Here's how the part is built. I have some questions about the finished solid (model axes, mm). Face numbers are marked on the shaded views. A direction names the side the tool comes from. Coordinates: 2 decimals unless noted, no trailing zeros. Write each loop counter-clockwise with the first axis right and the second up, starting at its lowest first coordinate (ties: lowest second). Pieces come first, ordered by that corner, then holes. Notation, with made-up numbers: (-8, 69.25) - (21, 69.25) arc R17 ccw to (21, 93.25) - close; hole circle Ø4 at (-28.5, 48). An arc over 180 degrees is marked (long way). Answer in a Markdown table with one row per item. Add a question column.
Item 1: If I drill on probe 1 along X at (y, z) = (13, -67); probe 2 along X at (y, z) = (25.75, -47); probe 3 along Z at (x, y) = (35, 24.5), over which ranges is the centre line in solid material (lowest first)? Write a range as from..to.
Item 2: I'm going to push flat-ended pins straight in: pin 1 (1.5 mm diameter, centred on x = 60.5, y = 16.5, fed in from -Z); pin 2 (12 mm diameter, centred on x = 5, z = -53, fed in from -Y); pin 3 (3 mm diameter, centred on x = 37.5, y = 9.5, fed in from -Z). Where does each tip first touch, or does it pass through?
Item 3: Which directions (+Z, -Z, +X, -X, +Y, -Y) give clear straight access to the entire face, cutting with the end or side of a thin tool? Please do the marked faces 4 and 5.
Item 4: Imagine slicing it at B-B (y = 1.75). Please give me the cut outline in (x, z).
Item 5: Imagine slicing it at C-C (x = 14). Please give me the cut outline in (y, z), plus the area to 3 significant figures.
Item 6: Imagine slicing it at A-A (z = -51). Please give me the cut outline in (x, y), plus the area to 3 significant figures.
Item 7: Imagine slicing it at D-D (z = -43). Please give me the cut outline in (x, y) (3 decimals).
Item 8: We'd pull the mould along X, two halves only. Please class the marked faces 1, 2 and 3: +X half, -X half, draft (parallel to the pull), parting line (faces both ways), or undercut.
from build123d import *

# Parameters (mm, degrees)
SKIZZE1_W                       = 95
SKIZZE1_H                       = 70
AUFSATZ_LINEAR_AUSTRAGEN1_DEPTH = 28.3
SCHNITT_LINEAR_AUSTRAGEN1_REACH = 123.35
SKIZZE2_W                       = 7.37
SKIZZE2_H                       = 3
SCHNITT_LINEAR_AUSTRAGEN2_DEPTH = 30
VERRUNDUNG1_R                   = 8.5
AUFSATZ_LINEAR_AUSTRAGEN3_DEPTH = 3
VERRUNDUNG2_R                   = 8


with BuildPart() as part:
    # Skizze1 → Aufsatz-Linear austragen1 (new body)
    with BuildSketch(Plane(origin=(0, 0, 0), x_dir=(1, 0, 0), z_dir=(0, 1, 0))):
        with Locations((47.5, 35)):
            Rectangle(SKIZZE1_W, SKIZZE1_H)
    extrude(amount=AUFSATZ_LINEAR_AUSTRAGEN1_DEPTH)

    # Skizze2 → Schnitt-Linear austragen1 (cut, up to next)
    with BuildSketch(Plane.XY, mode=Mode.PRIVATE) as schnitt_linear_austragen1_sk1:
        with Locations((58.855, 26.8)):
            Rectangle(SKIZZE2_W, SKIZZE2_H)
    schnitt_linear_austragen1_tool1 = extrude(schnitt_linear_austragen1_sk1.sketch, amount=-SCHNITT_LINEAR_AUSTRAGEN1_REACH, mode=Mode.PRIVATE) & part.part
    add(schnitt_linear_austragen1_tool1.solids().sort_by_distance((58.855, 26.8, 0))[0], mode=Mode.SUBTRACT)

    # Skizze4 → Schnitt-Linear austragen2 (cut)
    with BuildSketch(Plane(origin=(0, 0, -70), x_dir=(-1, 0, 0), z_dir=(0, 0, -1))):
        Polygon((-3.63, 0), (-71.13, 0), (-71.13, 3), (-66.63, 3), (-66.63, 28.3), (-49.63, 28.3), (-49.63, 3), (-43.63, 3), (-43.63, 28.3), (-26.63, 28.3), (-26.63, 3), (-20.63, 3), (-20.63, 28.3), (-3.63, 28.3), (-3.63, 3), (0, 3), (0, 0), align=None)
    extrude(amount=-SCHNITT_LINEAR_AUSTRAGEN2_DEPTH, mode=Mode.SUBTRACT)

    # Verrundung1
    verrundung1_edges = [part.edges().sort_by_distance(p)[0] for p in [
        (3.63, 15.65, -40),
        (20.63, 15.65, -40),
        (26.63, 15.65, -40),
        (43.63, 15.65, -40),
        (49.63, 15.65, -40),
        (66.63, 15.65, -40),
    ]]
    fillet(verrundung1_edges, radius=VERRUNDUNG1_R - 0.0001)  # a hair under: the kernel refuses the full size

    # Skizze5 → Aufsatz-Linear austragen3 (add)
    with BuildSketch(Plane.ZY):
        Polygon((0, 0), (-40, 0), (-40, 3), (-70, 3), (-70, 28.3), (0, 28.3), align=None)
    extrude(amount=AUFSATZ_LINEAR_AUSTRAGEN3_DEPTH)

    # Verrundung2
    verrundung2_edges = [part.edges().sort_by_distance(p)[0] for p in [
        (71.13, 1.5, -40),
    ]]
    fillet(verrundung2_edges, radius=VERRUNDUNG2_R)


solid = part.part
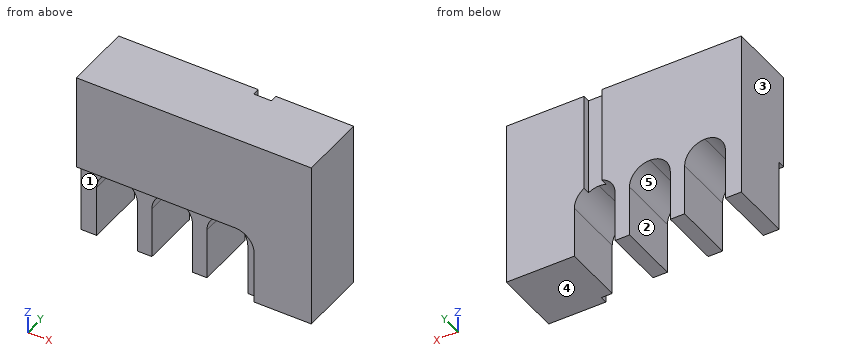
Here are the results:
| question | item | result |
|---|---|---|
| 1 | probe 1 | x = -3..3.63, 20.63..26.63, 43.63..49.63, 66.63..95 |
| 1 | probe 2 | x = -3..3.76, 20.5..26.76, 43.5..49.76, 66.5..95 |
| 1 | probe 3 | z = -40..0 |
| 2 | pin 1 | stops at z = -40.59 |
| 2 | pin 2 | stops at y = 3 |
| 2 | pin 3 | stops at z = -40.93 |
| 3 | face 4 | -Z, +X, -X, +Y, -Y |
| 3 | face 5 | -Z, +Y, -Y |
| 4 | outline | (-3, -40) - (63.13, -40) arc R8 cw to (71.13, -48) - (71.13, -70) - (95, -70) - (95, 0) - (-3, 0) - close |
| 5 | outline | (0, -40) - (3, -40) - (3, -40.21) - (28.3, -40.21) - (28.3, 0) - (0, 0) - close |
| 5 | area | 1,140 mm2 |
| 6 | outline | (-3, 3) - (3.63, 3) - (3.63, 28.3) - (-3, 28.3) - close; (20.63, 3) - (26.63, 3) - (26.63, 28.3) - (20.63, 28.3) - close; (43.63, 3) - (49.63, 3) - (49.63, 28.3) - (43.63, 28.3) - close; (66.63, 3) - (71.13, 3) - (71.13, 0) - (95, 0) - (95, 28.3) - (66.63, 28.3) - close |
| 6 | area | 1,260 mm2 |
| 7 | outline | (-3, 3) - (5.649, 3) - (5.649, 28.3) - (-3, 28.3) - close; (18.611, 3) - (28.649, 3) - (28.649, 28.3) - (18.611, 28.3) - close; (41.611, 3) - (51.649, 3) - (51.649, 28.3) - (41.611, 28.3) - close; (64.611, 3) - (69.375, 3) - (69.375, 0) - (95, 0) - (95, 28.3) - (64.611, 28.3) - close |
| 8 | face 1 | draft |
| 8 | face 2 | undercut |
| 8 | face 3 | -X half |
